```python
from build123d import *

# Parameters (mm, degrees)
F0_W     = 67
F0_H     = 21
F1_DEPTH = 70
F2_W     = 63.5
F2_H     = 17.5
F3_DEPTH = 68
F4_R     = 7.5
F4_W     = 25
F4_H     = 6
F5_DEPTH = 2
F6_R     = 4.5
F7_DEPTH = 21.001


with BuildPart() as f1:
    # F0 (on Top) → F1 (new body)
    with BuildSketch(Plane.XY):
        Rectangle(F0_W, F0_H)
    extrude(amount=F1_DEPTH)

    # F2 (on face) → F3 (cut)
    with BuildSketch(Plane.XY.offset(70)):
        Rectangle(F2_W, F2_H)
    extrude(amount=-F3_DEPTH, mode=Mode.SUBTRACT)

    # F4 (on face) → F5 (cut, through all)
    with BuildSketch(Plane(origin=(0, 0, 0), x_dir=(1, 0, 0), z_dir=(0, 0, -1))):
        with Locations((-23, 0)):
            Circle(F4_R)
        with Locations((23, 0)):
            Circle(F4_R)
        with Locations((0, 5.5)):
            Rectangle(F4_W, F4_H)
        with Locations((0, -5.5)):
            Rectangle(F4_W, F4_H)
    extrude(amount=-F5_DEPTH, mode=Mode.SUBTRACT)

    # F6 (on face) → F7 (cut, through all)
    with BuildSketch(Plane(origin=(0, 10.5, 0), x_dir=(-1, 0, 0), z_dir=(0, 1, 0))):
        with Locations((24, 60)):
            Circle(F6_R)
        with Locations((24, 48)):
            Circle(F6_R)
        with Locations((24, 36)):
            Circle(F6_R)
        with Locations((24, 24)):
            Circle(F6_R)
        with Locations((24, 12)):
            Circle(F6_R)
        with Locations((12, 60)):
            Circle(F6_R)
        with Locations((12, 48)):
            Circle(F6_R)
        with Locations((12, 36)):
            Circle(F6_R)
        with Locations((12, 24)):
            Circle(F6_R)
        with Locations((12, 12)):
            Circle(F6_R)
        with Locations((0, 60)):
            Circle(F6_R)
        with Locations((0, 48)):
            Circle(F6_R)
        with Locations((0, 36)):
            Circle(F6_R)
        with Locations((0, 24)):
            Circle(F6_R)
        with Locations((0, 12)):
            Circle(F6_R)
        with Locations((-12, 60)):
            Circle(F6_R)
        with Locations((-12, 48)):
            Circle(F6_R)
        with Locations((-12, 36)):
            Circle(F6_R)
        with Locations((-12, 24)):
            Circle(F6_R)
        with Locations((-12, 12)):
            Circle(F6_R)
        with Locations((-24, 60)):
            Circle(F6_R)
        with Locations((-24, 48)):
            Circle(F6_R)
        with Locations((-24, 36)):
            Circle(F6_R)
        with Locations((-24, 24)):
            Circle(F6_R)
        with Locations((-24, 12)):
            Circle(F6_R)
    extrude(amount=-F7_DEPTH, mode=Mode.SUBTRACT)


solid = f1.part
```
Work out the finished part from the listing and answer in its coordinate system (mm). A direction names the side the tool comes from. Round coordinates to 2 decimals unless told otherwise and drop trailing zeros. Loops run counter-clockwise (first coordinate to the right, second up) from the corner with the lowest first, then second, coordinate; pieces in that order, holes last. Notation, with made-up numbers: M -23,40.5 L 6,40.5 A24 ccw 6,69.5 Z; hole C -21.75,76.25 d5. An arc over 180 degrees is marked long. One line per question, with ' | ' between items.
Q1. Consider line 1 along Z through (x, y) = (0, 9.15); line 2 along X through (y, z) = (-8.25, 49); line 3 along Y through (x, z) = (9, 5). Determine where each line is inside the solid, lowest interval first. Write a range as from..to.
Conclusion:
line 1: z = 0..7.5, 16.5..19.5, 28.5..31.5, 40.5..43.5, 52.5..55.5, 64.5..70 | line 2: x = -33.5..-31.75, 31.75..33.5 | line 3: y = -10.5..-8.75, 8.75..10.5
Q2. Find section B-B, the plane z = 48. State how many separate pieces and enclosed holes the cut face has, then the cut area to 3 significant figures.
Conclusion:
separate pieces: 10 | enclosed holes: 0 | area: 138 mm2
Q3. The mould has two halves that part along X. Classify faces 1 (the flat face through (33.5, 0, 35)), 2 (the cylindrical face through (0.98, 9.64, 43.61)): +X half, -X half, draft (parallel to the pull), parting line (faces both ways), or undercut.
Conclusion:
face 1: +X half | face 2: undercut
Q4. Each of these flat-tipped pins is pushed along its axis until it touches: pin 1 Ø6 at (x, y) = (16, -1) entering from +Z; pin 2 Ø10.5 at (x, z) = (24, 24) entering from -Y. Where does it stop, or does it pass through?
Conclusion:
pin 1: stops at z = 2 | pin 2: stops at y = -10.5
Q5. Find section A-A, the plane y = 5.25. Give the vertices of the cut face in (x, z).
Conclusion:
outline: M -33.5,0 L -28.36,0 L -28.36,2 L -31.75,2 L -31.75,70 L -33.5,70 Z; M -17.64,0 L -12.5,0 L -12.5,2 L -17.64,2 Z; M 12.5,0 L 17.64,0 L 17.64,2 L 12.5,2 Z; M 28.36,0 L 33.5,0 L 33.5,70 L 31.75,70 L 31.75,2 L 28.36,2 Z
Q6. A tool of negligible diameter and unlimited length cuts with its end or side. For faces 3 (the cylindrical face through (24.98, -9.61, 43.61)), 4 (the flat face through (-12.5, -5, 1)), from which of +Z, -Z, +X, -X, +Y, -Y can it reach the whole face along a straight path? Write none if from no direction.
Conclusion:
face 3: +Y, -Y | face 4: +Z, -Z
